The model under review builds one solid part; all positions refer to its coordinate system, in mm. A direction names the side the tool comes from. Give positions to 0.01 mm unless a question says otherwise; leave off trailing zeros. Order: outer loops, then holes, each group sorted by start corner. A loop starts at its lowest first (then second) coordinate and runs counter-clockwise, first axis right, second up. Notation, with made-up numbers: (31, 8.5) -> (54, 8.5) arc R13 cw to (54, 30.5) -> close; hole circle Ø5 at (10, 28.5). An arc over 180 degrees is marked (long way). Use one line per item in the form item = value.
Autodesk Inventor part; units mm, degrees
ref_plane "YZ Plane" through (0, 0, 0) normal (1, 0, 0) x (0, 1, 0)
ref_plane "XZ Plane" through (0, 0, 0) normal (0, 1, 0) x (-1, 0, 0)
ref_plane "XY Plane" through (0, 0, 0) normal (0, 0, 1) x (1, 0, 0)
sketch "Sketch1" plane through (0, 0, 0) normal (0, 1, 0) x (-1, 0, 0)
  line L0 (0, 0) -> (-25.4, 0)
  line L1 (-25.4, 0) -> (-25.4, 50.8)
  line L2 (-25.4, 50.8) -> (0, 50.8)
  line L3 (0, 50.8) -> (0, 0)
  line L4 (-3.175, 3.175) -> (-22.225, 3.175)
  line L5 (-22.225, 3.175) -> (-22.225, 47.625)
  line L6 (-22.225, 47.625) -> (-3.175, 47.625)
  line L7 (-3.175, 47.625) -> (-3.175, 3.175)
  dimension "d0" = 25.4
  dimension "d1" = 50.8
  dimension "d2" = 3.175
extrude "Extrusion1" add sketch "Sketch1" along normal blind 355.6
sketch "Sketch2" plane through (25.4, 0, 50.8) normal (1, 0, 0) x (0, 0, -1)
  circle A0 centre (25.4, 25.4) radius 14.2875
  line L0 (50.8, 0) -> (50.8, 355.6)
  line L1 (50.8, 0) -> (0, 0)
  dimension "d5" = 28.575
  dimension "d6" = 25.4
  dimension "d7" = 25.4
extrude "Extrusion2" cut sketch "Sketch2" against normal blind 25.4
sketch "Sketch3" plane through (0, 0, 0) normal (-1, 0, 0) x (0, 0, 1)
  line L0 (50.8, 0) -> (50.8, 355.6)
  line L1 (0, 355.6) -> (50.8, 355.6)
  line L2 (0, 0) -> (0, 355.6)
  line L3 (0, 0) -> (50.8, 0)
  point P0 (38.1, 346.075)
  point P1 (38.1, 190.5)
  point P2 (38.1, 320.675)
  point P3 (12.7, 215.9)
  dimension "d10" = 12.7
  dimension "d11" = 9.525
  dimension "d19" = 25.4
  dimension "d20" = 38.1
  dimension "d21" = 38.1
  dimension "d23" = 190.5
  dimension "d26" = 215.9
  dimension "d27" = 12.7
hole "Hole1" at (0, 346.075, 38.1) at (0, 320.675, 38.1) at (0, 190.5, 38.1) at (0, 215.9, 12.7) direction (1, 0, 0) diameter 6.35 end through all
sketch "Sketch4" plane through (0, 0, 0) normal (-1, 0, 0) x (0, 0, 1)
  line L0 (0, 0) -> (0, 355.6)
  line L1 (25.4, 355.6) -> (0, 355.6)
  line L2 (0, 355.6) -> (0, 254)
  line L3 (0, 254) -> (25.4, 254)
  line L4 (25.4, 254) -> (25.4, 355.6)
  line L5 (0, 355.6) -> (50.8, 355.6)
  line L6 (50.8, 0) -> (50.8, 355.6)
  line L7 (50.8, 0) -> (0, 0)
  dimension "d28" = 25.4
  dimension "d29" = 254
extrude "Extrusion3" cut sketch "Sketch4" against normal blind 25.4 contours L0 L1 L4 L3
sketch "Sketch6" plane through (25.4, 0, 50.8) normal (1, 0, 0) x (0, 0, -1)
  line L0 (50.8, 0) -> (50.8, 254)
  line L1 (50.8, 19.05) -> (39.8015, 0)
  line L2 (3.175, 0) -> (47.625, 0)
  line L3 (50.8, 0) -> (0, 0)
  line L4 (47.625, 0) -> (50.8, 0)
  dimension "d52" = 30
  dimension "d53" = 9.525
extrude "Extrusion5" cut sketch "Sketch6" against normal blind 25.4
equation "\"BendRadius\" = Thickness"
equation "\"BendReliefWidth\" = Thickness"
equation "\"BendReliefDepth\" = 0.5 * Thickness"
equation "\"CornerReliefSize\" = 4 * Thickness"
equation "\"MinimumRemnant\" = 2 * Thickness"
equation "\"TransitionRadius\" = BendRadius"
equation "\"JacobiRadiusSize\" = Thickness"
equation "\"GapSize\" = Thickness"
properties part number "15102898-16-A-0301" material "Aluminum 6061"
1. The part is to be moulded in two halves that separate along Z. For faces 1 (the face through (0, 175, 31)), 2 (the face through (13, 132, 3.175)), 3 (the face through (12.88, 13.89, 2.98)), say which applies: +Z half, -Z half, draft (parallel to the pull), parting line (faces both ways), or undercut.
Values:
face_1 = draft
face_2 = undercut
face_3 = -Z half
2. Add section A-A on y = 190.5. Give the boundary of the cut face in (x, z) (3 decimals).
Values:
outline = (0, 0) -> (25.4, 0) -> (25.4, 34.925) -> (22.225, 34.925) -> (22.225, 3.175) -> (3.175, 3.175) -> (3.175, 34.925) -> (0, 34.925) -> close; (0, 41.275) -> (3.175, 41.275) -> (3.175, 47.625) -> (22.225, 47.625) -> (22.225, 41.275) -> (25.4, 41.275) -> (25.4, 50.8) -> (0, 50.8) -> close
3. Add section D-D on z = 19. Give the boundary of the cut face in (x, y) (3 decimals), then the cut area to 3 significant figures.
Values:
outline = (0, 0) -> (3.175, 0) -> (3.175, 12.626) -> (0, 12.626) -> close; (0, 38.174) -> (3.175, 38.174) -> (3.175, 254) -> (0, 254) -> close; (22.225, 0) -> (25.4, 0) -> (25.4, 12.626) -> (22.225, 12.626) -> close; (22.225, 38.174) -> (25.4, 38.174) -> (25.4, 254) -> (22.225, 254) -> close
area = 1,450 mm^2
4. Tool access review of faces 4 (the face through (13, 254, 2)), 5 (the face through (13, 135, 0)), 6 (the face through (13, 175, 47.625)): name each direction out of +Z, -Z, +X, -X, +Y, -Y from which nothing blocks a thin tool from reaching the whole face with its end or side.
Values:
face_4 = -Z, +X, -X, +Y
face_5 = -Z, +X, -X, +Y, -Y
face_6 = +Y, -Y
5. For pin 1 Ø3 at (x, z) = (19.5, 20.5) entering from +Y; pin 2 Ø8 at (y, z) = (270.5, 34) entering from -X; pin 3 Ø1 at (x, y) = (1.5, 298) entering from -Z; pin 4 Ø1 at (x, z) = (22.5, 9) entering from -Y, all flat-tipped, find the tip position at first contact; note any pin that passes through.
Values:
pin_1 = through
pin_2 = 0
pin_3 = 25.4
pin_4 = 2.6
6. Add section C-C on x = 10.75. Give the boundary of the cut face in (y, z) (3 decimals).
Values:
outline = (0, 47.625) -> (355.6, 47.625) -> (355.6, 50.8) -> (0, 50.8) -> close; (13.551, 3.175) -> (19.05, 0) -> (254, 0) -> (254, 3.175) -> close
7. Add section B-B on y = 87. Give the boundary of the cut face in (x, z) (3 decimals).
Values:
outline = (0, 0) -> (25.4, 0) -> (25.4, 50.8) -> (0, 50.8) -> close; hole (3.175, 3.175) -> (22.225, 3.175) -> (22.225, 47.625) -> (3.175, 47.625) -> close
8. For L1, parallel to Z at x = 18.25, y = 185.5 (3 decimals); L2, parallel to X at y = 332.5, z = 40.5 (3 decimals); L3, parallel to Z at x = 24.05, y = 190.5 (3 decimals), list the stretches that pass through material, from the lowest coordinate up.
Values:
L1 = 0 to 3.175, 47.625 to 50.8
L2 = 0 to 3.175, 22.225 to 25.4
L3 = 0 to 34.925, 41.275 to 50.8
